The listing builds one solid part. Answer for the finished solid, in the listing's coordinates (mm). Face numbers are marked on the shaded views. Coordinates: 2 decimals unless noted, no trailing zeros. Loops run counter-clockwise (first coordinate to the right, second up) from the corner with the lowest first, then second, coordinate; pieces in that order, holes last. Notation, with made-up numbers: (83, 16.25) - (116, 16.25) arc R17 cw to (116, 29.25) - close; hole circle Ø3 at (46.25, 10). An arc over 180 degrees is marked (long way). Put each result on its own line as item: value.
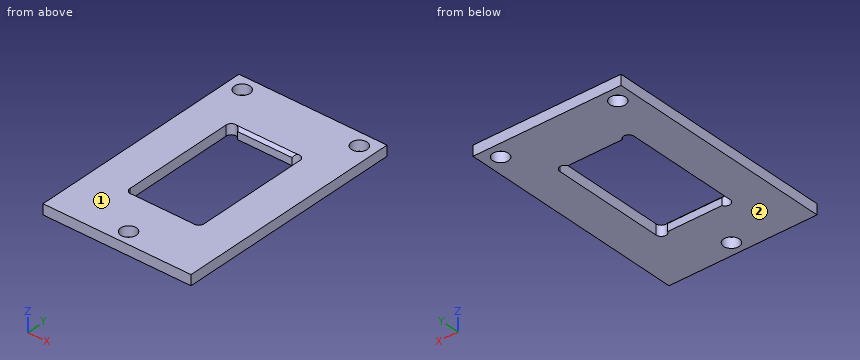
```python
from build123d import *

# Parameters (mm, degrees)
F0_W     = 45.72
F0_H     = 71.12
F0_R     = 2.413
F1_DEPTH = 3.175
F2_SIZE  = 0.889


with BuildPart() as f1:
    # F0 (on Top) → F1 (new body)
    with BuildSketch(Plane.XY):
        Rectangle(F0_W, F0_H)
        with Locations((0, -31.369)):
            Circle(F0_R, mode=Mode.SUBTRACT)
        with BuildLine():
            ThreePointArc((11.43, -17.4625), (10.166842, -19.016514), (8.387532, -18.0975))
            Line((8.387532, -18.0975), (-8.387532, -18.0975))
            ThreePointArc((-8.387532, -18.0975), (-10.166842, -19.016514), (-11.43, -17.4625))
            Line((-11.43, -17.4625), (-11.43, 17.4625))
            ThreePointArc((-11.43, 17.4625), (-10.166842, 19.016514), (-8.387532, 18.0975))
            Line((-8.387532, 18.0975), (8.387532, 18.0975))
            ThreePointArc((8.387532, 18.0975), (10.166842, 19.016514), (11.43, 17.4625))
            Line((11.43, 17.4625), (11.43, -17.4625))
        make_face(mode=Mode.SUBTRACT)
        with Locations((-18.0975, 31.115)):
            Circle(F0_R, mode=Mode.SUBTRACT)
        with Locations((18.0975, 31.115)):
            Circle(F0_R, mode=Mode.SUBTRACT)
    extrude(amount=F1_DEPTH)

    # F2
    f2_edges = [f1.edges().sort_by_distance(p)[0] for p in [
        (0, 18.0975, 3.175),
        (0, -18.0975, 3.175),
    ]]
    chamfer(f2_edges, length=F2_SIZE)


solid = f1.part
```
1) The part is cut by section A-A (y = -7.5). Give the vertices of the cut face in (x, z) (3 decimals), and give its area (3 significant figures).
Found:
outline: (-22.86, 0) - (-11.43, 0) - (-11.43, 3.175) - (-22.86, 3.175) - close; (11.43, 0) - (22.86, 0) - (22.86, 3.175) - (11.43, 3.175) - close
area: 72.6 mm^2
2) The part is cut by section B-B (x = 0). Give the vertices of the cut face in (y, z) (1 decimal), and give its area (3 significant figures).
Found:
outline: (-35.6, 0) - (-33.8, 0) - (-33.8, 3.2) - (-35.6, 3.2) - close; (-29, 0) - (-18.1, 0) - (-18.1, 2.3) - (-19, 3.2) - (-29, 3.2) - close; (18.1, 0) - (35.6, 0) - (35.6, 3.2) - (19, 3.2) - (18.1, 2.3) - close
area: 94.8 mm^2
3) Straight lines are drawn through the part: L1, parallel to X at y = 10, z = 0.3; L2, parallel to Y at x = 10, z = 1.7; L3, parallel to X at y = 32, z = 1.7. For each, find the intervals that lie inside material, in ascending order. Write a range as [from, to].
Found:
L1: x = [-22.86, -11.43], [11.43, 22.86]
L2: y = [-35.56, -19.04], [19.04, 35.56]
L3: x = [-22.86, -20.34], [-15.85, 15.85], [20.34, 22.86]
4) The part is cut by section D-D (y = 30). Give the vertices of the cut face in (x, z) (3 decimals), and give its area (3 significant figures).
Found:
outline: (-22.86, 0) - (-20.237, 0) - (-20.237, 3.175) - (-22.86, 3.175) - close; (-15.958, 0) - (15.958, 0) - (15.958, 3.175) - (-15.958, 3.175) - close; (20.237, 0) - (22.86, 0) - (22.86, 3.175) - (20.237, 3.175) - close
area: 118 mm^2
5) For a pull along Z with two mould halves and no side action, classify the marked faces 1 and 2 as pulls with the +Z half, pulls with the -Z half, needs draft (parallel to the pull), parting line crosses it, or undercut.
Found:
face 1: pulls with the +Z half
face 2: pulls with the -Z half
6) The part is cut by section C-C (x = -19). Give the vertices of the cut face in (y, z) (3 decimals), and give its area (3 significant figures).
Found:
outline: (-35.56, 0) - (28.877, 0) - (28.877, 3.175) - (-35.56, 3.175) - close; (33.353, 0) - (35.56, 0) - (35.56, 3.175) - (33.353, 3.175) - close
area: 212 mm^2
